Check sheet for the drawn part. Datum: minimum x, y, z corner. Units: mm. Coordinates: 2 decimals unless noted, no trailing zeros. Write each loop counter-clockwise with the first axis right and the second up, starting at its lowest first coordinate (ties: lowest second). Pieces come first, ordered by that corner, then holes. Notation, with made-up numbers: (8.5, -12.75) - (48.5, -12.75) arc R12 ccw to (48.5, -7.75) - close; hole circle Ø11 at (-31, -25.75). An arc over 180 degrees is marked (long way). Use one line per item in the form item = value. Start each with the question number.
1. Cross-section at C-C on z = 2.1. Record the boundary of the cut face in (x, y).
2. Scan lines: line 1 along Y through (x, z) = (18.5, 0.45); line 2 along Y through (x, z) = (44, 1.5) (1 decimal); line 3 along X through (y, z) = (51, 0.8). Record each from-to range of solid material in increasing order.
3. Cross-section at D-D on y = 10.5. Record the boundary of the cut face in (x, z) (1 decimal).
4. Cross-section at A-A on x = 49.5. Record the boundary of the cut face in (y, z) (1 decimal), then the cut area to 3 significant figures.
5. Cross-section at B-B on y = 53. Record the boundary of the cut face in (x, z) (1 decimal).
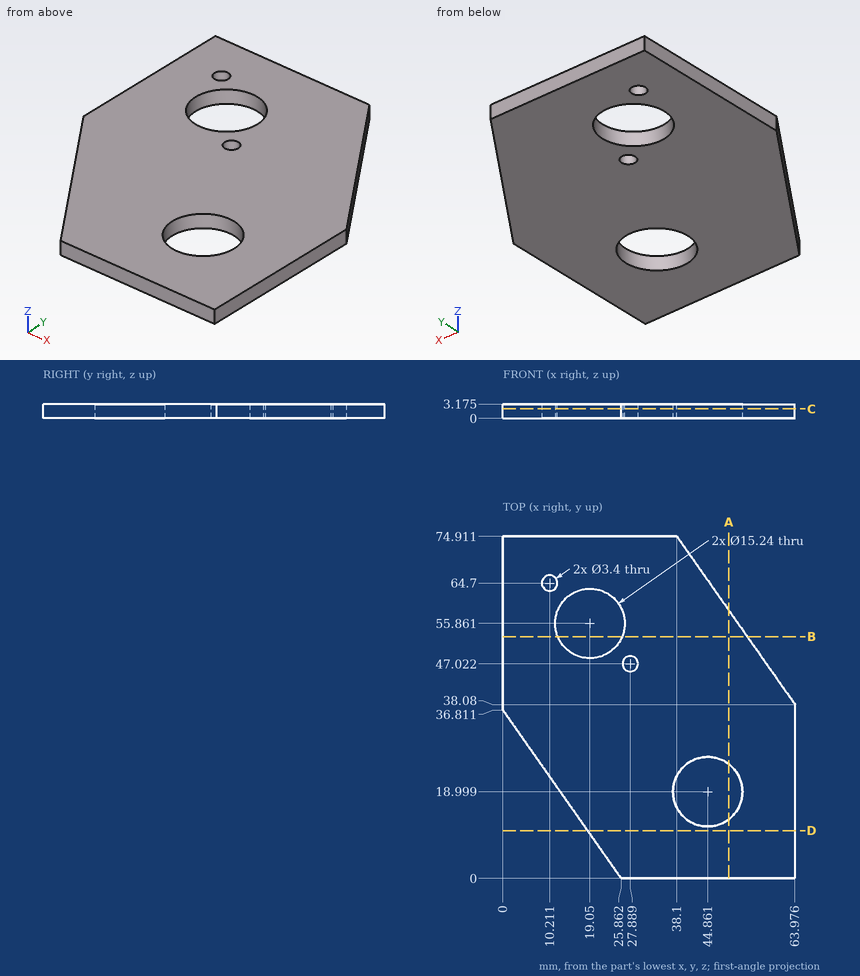
Final values:
q1.outline = (0, 36.81) - (25.86, 0) - (63.98, 0) - (63.98, 38.08) - (38.1, 74.91) - (0, 74.91) - close; hole circle Ø3.4 at (10.21, 64.7); hole circle Ø15.24 at (19.05, 55.86); hole circle Ø3.4 at (27.89, 47.02); hole circle Ø15.24 at (44.86, 19)
q2.line_1 = 10.48 to 48.26, 63.46 to 74.91
q2.line_2 = 0 to 11.4, 26.6 to 66.5
q2.line_3 = 0 to 13.18, 24.92 to 54.9
q3.outline = (18.5, 0) - (64, 0) - (64, 3.2) - (18.5, 3.2) - close
q4.outline = (0, 0) - (13, 0) - (13, 3.2) - (0, 3.2) - close; (25, 0) - (58.7, 0) - (58.7, 3.2) - (25, 3.2) - close
q4.area = 148 mm²
q5.outline = (0, 0) - (12, 0) - (12, 3.2) - (0, 3.2) - close; (26.1, 0) - (53.5, 0) - (53.5, 3.2) - (26.1, 3.2) - close
